Geometry check sheet. Reference: the model listing, model coordinates, mm. A direction names the side the tool comes from. Give positions to 0.01 mm unless a question says otherwise; leave off trailing zeros. Order: outer loops, then holes, each group sorted by start corner. A loop starts at its lowest first (then second) coordinate and runs counter-clockwise, first axis right, second up. Notation, with made-up numbers: (19, 36) - (27, 36) arc R23 ccw to (27, 64) - close; hole circle Ø10 at (81.5, -8.5). An arc over 180 degrees is marked (long way). Put each result on its own line as item: value. Start each with the question number.
```python
from build123d import *

# Parameters (mm, degrees)
EXTRUDE_3_DEPTH      = 22.5
EXTRUDE_3_DEPTH_BACK = 22.5
FILLET_3_R           = 2.5
SKETCH_6_W           = 42
SKETCH_6_H           = 87
CUT_EXTRUDE_2_DEPTH  = 1
EXTRUDE_5_DEPTH      = 10
SKETCH_9_W           = 10
SKETCH_9_H           = 1.4
EXTRUDE_6_DEPTH      = 1.5
FILLET_4_R           = 1


with BuildPart() as part:
    # Sketch 3 → Extrude 3 (new body, two sides)
    with BuildSketch(Plane.XY) as extrude_3_sk:
        with BuildLine():
            Line((0.5, -45), (2, -45))
            Line((2, -45), (2, 45))
            Line((2, 45), (0.5, 45))
            ThreePointArc((0.5, 45), (-1.267766953, 44.267766953), (-2, 42.5))
            Line((-2, 42.5), (-2, -42.5))
            ThreePointArc((-2, -42.5), (-1.267766953, -44.267766953), (0.5, -45))
        make_face()
    extrude(amount=EXTRUDE_3_DEPTH)
    extrude(extrude_3_sk.sketch, amount=-EXTRUDE_3_DEPTH_BACK)

    # Fillet 3
    fillet_3_edges = [part.edges().sort_by_distance(p)[0] for p in [
        (-1.267766953, 44.267766953, -22.5),
        (-2, 0, -22.5),
        (1.25, 45, 22.5),
        (-1.267766953, 44.267766953, 22.5),
        (-2, 0, 22.5),
        (-1.267766953, -44.267766953, 22.5),
        (1.25, -45, 22.5),
        (-1.267766953, -44.267766953, -22.5),
        (1.25, -45, -22.5),
        (1.25, 45, -22.5),
    ]]
    fillet(fillet_3_edges, radius=FILLET_3_R)

    # Sketch 6 → Cut-Extrude 2 (cut)
    with BuildSketch(Plane(origin=(2, 0, 0), x_dir=(0, 0, -1), z_dir=(1, 0, 0))):
        Rectangle(SKETCH_6_W, SKETCH_6_H)
    extrude(amount=-CUT_EXTRUDE_2_DEPTH, mode=Mode.SUBTRACT)

    # Sketch 7 → Extrude 5 (add)
    with BuildSketch(Plane(origin=(1, 0, 0), x_dir=(0, 0, -1), z_dir=(1, 0, 0))):
        with BuildLine():
            Line((-0.5, 22.474937186), (-0.5, 20.964101615))
            ThreePointArc((-0.5, 20.964101615), (-3.5, 17.5), (-0.5, 14.035898385))
            Line((-0.5, 14.035898385), (-0.5, 12.525062814))
            ThreePointArc((-0.5, 12.525062814), (-5, 17.5), (-0.5, 22.474937186))
        make_face()
        with BuildLine():
            Line((0.5, 22.474937186), (0.5, 20.964101615))
            ThreePointArc((0.5, 20.964101615), (3.5, 17.5), (0.5, 14.035898385))
            Line((0.5, 14.035898385), (0.5, 12.525062814))
            ThreePointArc((0.5, 12.525062814), (5, 17.5), (0.5, 22.474937186))
        make_face()
        with BuildLine():
            Line((-0.5, -14.035898385), (-0.5, -12.525062814))
            ThreePointArc((-0.5, -12.525062814), (-5, -17.5), (-0.5, -22.474937186))
            Line((-0.5, -22.474937186), (-0.5, -20.964101615))
            ThreePointArc((-0.5, -20.964101615), (-3.5, -17.5), (-0.5, -14.035898385))
        make_face()
        with BuildLine():
            Line((0.5, -14.035898385), (0.5, -12.525062814))
            ThreePointArc((0.5, -12.525062814), (5, -17.5), (0.5, -22.474937186))
            Line((0.5, -22.474937186), (0.5, -20.964101615))
            ThreePointArc((0.5, -20.964101615), (3.5, -17.5), (0.5, -14.035898385))
        make_face()
    extrude(amount=EXTRUDE_5_DEPTH)

    # Sketch 9 → Extrude 6 (add)
    with BuildSketch(Plane(origin=(2, 0, 0), x_dir=(0, 0, -1), z_dir=(1, 0, 0))):
        with Locations((0, -44.2)):
            Rectangle(SKETCH_9_W, SKETCH_9_H)
    extrude(amount=EXTRUDE_6_DEPTH)

    # Fillet 4
    fillet_4_edges = [part.edges().sort_by_distance(p)[0] for p in [
        (3.5, -44.2, 5),
        (3.5, -44.2, -5),
    ]]
    fillet(fillet_4_edges, radius=FILLET_4_R)


solid = part.part
```
Item 1: Set-up check for faces 4 (the face through (5.9, 17.6, 3.5)), 5 (the face through (11, 18, 4)): record each of +Z, -Z, +X, -X, +Y, -Y from which the full face is reachable in a straight line by a thin tool's end or side.
Item 2: Release check for a two-part mould opening along Y. For faces 1 (the face through (-2, 1, 0)), 2 (the face through (5.9, 17.6, -3.5)), 3 (the face through (1, 44, 22)) record: +Y half, -Y half, draft (parallel to the pull), parting line (faces both ways), or undercut.
Item 3: Cross-section at A-A (y = 11). Enter the section's corners in (x, z), and give its area (3 significant figures).
Item 4: Gauge pin test, flat ends, axial feed: pin 1 Ø0.5 at (x, y) = (6.5, 13) entering from +Z; pin 2 Ø1.5 at (x, y) = (5.5, 15) entering from +Z; pin 3 Ø1.2 at (x, y) = (5.5, -22) entering from -Z. Record the tip position at first contact, or that the pin passes through.
Item 5: Cross-section at B-B (x = 5.5). Enter the section's corners in (y, z).
Item 6: Cross-section at D-D (x = -0.75). Enter the section's corners in (y, z).
Item 7: Cross-section at C-C (z = -12). Enter the section's corners in (x, y), and give its area (3 significant figures).
Item 8: Thickness scan on line 1 along Z through (x, y) = (1.75, 5); line 2 along X through (y, z) = (38, 0.5); line 3 along Y through (x, z) = (2.5, 2). Record the ranges inside material, lowest first.
Recorded:
1. face 4: +X
1. face 5: +Z, -Z, +X, +Y, -Y
2. face 1: draft
2. face 2: undercut
2. face 3: +Y half
3. outline: (-2, -20) arc R2.5 ccw to (0.5, -22.5) - (2, -22.5) - (2, -21) - (1, -21) - (1, 21) - (2, 21) - (2, 22.5) - (0.5, 22.5) arc R2.5 ccw to (-2, 20) - close
3. area: 135 mm^2
4. pin 1: stops at z = 2.63
4. pin 2: stops at z = 4.68
4. pin 3: stops at z = -3.13
5. outline: (-22.47, -0.5) arc R5 ccw to (-12.53, -0.5) - (-14.04, -0.5) arc R3.5 cw to (-20.96, -0.5) - close; (-22.47, 0.5) - (-20.96, 0.5) arc R3.5 cw to (-14.04, 0.5) - (-12.53, 0.5) arc R5 ccw to start; (12.53, -0.5) arc R5 ccw to (22.47, -0.5) - (20.96, -0.5) arc R3.5 cw to (14.04, -0.5) - close; (12.53, 0.5) - (14.04, 0.5) arc R3.5 cw to (20.96, 0.5) - (22.47, 0.5) arc R5 ccw to start
6. outline: (-44.67, -20) arc R2.17 ccw to (-42.5, -22.17) - (42.5, -22.17) arc R2.17 ccw to (44.67, -20) - (44.67, 20) arc R2.17 ccw to (42.5, 22.17) - (-42.5, 22.17) arc R2.17 ccw to (-44.67, 20) - close
7. outline: (-2, -42.5) arc R2.5 ccw to (0.5, -45) - (2, -45) - (2, -43.5) - (1, -43.5) - (1, 43.5) - (2, 43.5) - (2, 45) - (0.5, 45) arc R2.5 ccw to (-2, 42.5) - close
7. area: 270 mm^2
8. line 1: z = -22.5 to -21, 21 to 22.5
8. line 2: x = -2 to 1
8. line 3: y = -44.9 to -43.5, -22.08 to -20.37, -14.63 to -12.92, 12.92 to 14.63, 20.37 to 22.08
